Could you check a few things on this model? Use its own coordinates, in mm. Face numbers are marked on the shaded views. A direction names the side the tool comes from. Give positions to 0.01 mm unless a question says otherwise; leave off trailing zeros. Order: outer loops, then holes, each group sorted by start corner. A loop starts at its lowest first (then second) coordinate and runs counter-clockwise, first axis right, second up. Notation, with made-up numbers: M -34.5,17 L 22.5,17 A15 cw 22.5,31 Z; hole C 85.25,64.25 d10. An arc over 180 degrees is marked long. Answer in a Markdown table with one row per item. Add a question column.
```python
from build123d import *

# Parameters (mm, degrees)
PAD004_DEPTH    = 5
POCKET004_DEPTH = 2.001
PAD005_DEPTH    = 15
SKETCH015_R     = 1.55
POCKET005_DEPTH = 5.001
POCKET006_DEPTH = 2.65


with BuildPart() as part:
    # Sketch013 → Pad004 (new body)
    with BuildSketch(Plane.XY):
        with BuildLine():
            ThreePointArc((0, -7.5), (7.5, 0), (0, 7.5))
            Line((0, 7.5), (-40, 7.5))
            Line((-40, 7.5), (-40, 3.25))
            Line((0, 3.25), (-40, 3.25))
            ThreePointArc((0, -3.25), (3.25, 0), (0, 3.25))
            Line((0, -3.25), (-40, -3.25))
            Line((-40, -3.25), (-40, -7.5))
            Line((0, -7.5), (-40, -7.5))
        make_face()
    extrude(amount=PAD004_DEPTH)

    # Sketch012 → Pocket004 (cut, through all)
    with BuildSketch(Plane.XY.offset(3)):
        with BuildLine():
            ThreePointArc((0, -5.5), (5.5, 0), (0, 5.5))
            Line((0, 5.5), (-40, 5.5))
            ThreePointArc((-40, 5.5), (-45.5, 0), (-40, -5.5))
            Line((0, -5.5), (-40, -5.5))
        make_face()
    extrude(amount=POCKET004_DEPTH, mode=Mode.SUBTRACT)

    # Sketch014 → Pad005 (join)
    with BuildSketch(Plane.XZ.offset(7.5)):
        Polygon((-49, 5), (-50, 4), (-50, 1.3), (-40, 1.3), (-40, 0), (-39, 0), (-39, 5), (-40, 5), align=None)
    extrude(amount=-PAD005_DEPTH)

    # Sketch015 → Pocket005 (cut, through all)
    with BuildSketch(Plane.XY):
        with Locations((-44.5, 0)):
            Circle(SKETCH015_R)
    extrude(amount=POCKET005_DEPTH, mode=Mode.SUBTRACT)

    # Sketch016 → Pocket006 (cut)
    with BuildSketch(Plane.XY.offset(1.8)):
        Polygon((-44.5, 3.3), (-47.357884, 1.65), (-47.357884, -1.65), (-47.357884, -8.65), (-41.642116, -8.65), (-41.642116, -1.65), (-41.642116, 1.65), align=None)
    extrude(amount=POCKET006_DEPTH, mode=Mode.SUBTRACT)


solid = part.part
```
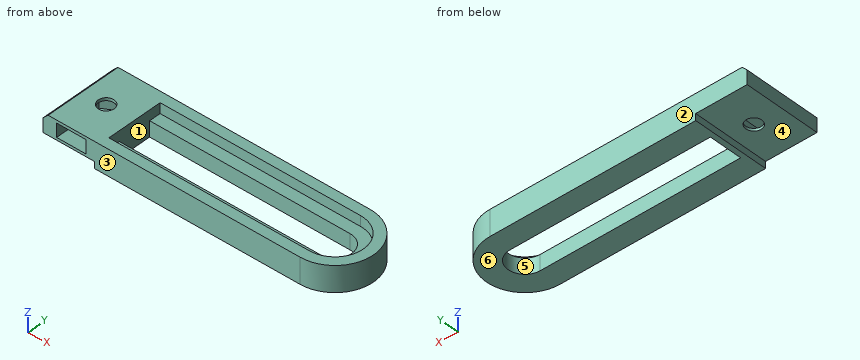
1. For the marked faces 4, 5 and 6, which set-ups out of +Z, -Z, +X, -X, +Y, -Y let a thin tool reach every point of the face, with its end or its side?
2. Suppose I cut it at A-A on x = -4. List the corners of the cut face in (y, z) for me, plus the area to 3 significant figures.
3. Suppose I cut it at B-B on y = 0. List the corners of the cut face in (x, z) for me, plus the area to 3 significant figures.
4. Thinking about a two-plate mould opening in Y: for the marked faces 1, 2 and 3, which applies, pulls with the +Y half, pulls with the -Y half, needs draft (parallel to the pull), parting line crosses it, or undercut?
5. If I drill on line 1 along Y through (x, z) = (-6.5, 3.45); line 2 along Y through (x, z) = (-44.5, 4.8); line 3 along X through (y, z) = (0, 4.85), over which ranges is the centre line in solid material (lowest first)? Write a range as [from, to].
6. Suppose I cut it at C-C on y = 4.75. List the corners of the cut face in (x, z) for me.
7. Will these pins go through, and if not, where does the flat tip stop? P1, Ø5, axis at x = -46.5, y = 3.5, coming from the -Z side; P2, Ø1.5, axis at y = 2.5, z = 3.5, coming from the +X side.
Findings below:
| question | item | result |
|---|---|---|
| 1 | face 4 | -Z, -X, +Y, -Y |
| 1 | face 5 | +Z, -Z |
| 1 | face 6 | -Z, +X, -X, +Y, -Y |
| 2 | outline | M -7.5,0 L -3.25,0 L -3.25,3 L -5.5,3 L -5.5,5 L -7.5,5 Z; M 3.25,0 L 7.5,0 L 7.5,5 L 5.5,5 L 5.5,3 L 3.25,3 Z |
| 2 | area | 33.5 mm2 |
| 3 | outline | M -50,1.3 L -46.05,1.3 L -46.05,1.8 L -47.36,1.8 L -47.36,4.45 L -46.05,4.45 L -46.05,5 L -49,5 L -50,4 Z; M -42.95,1.3 L -40,1.3 L -40,0 L -39,0 L -39,5 L -42.95,5 L -42.95,4.45 L -41.64,4.45 L -41.64,1.8 L -42.95,1.8 Z; M 3.25,0 L 7.5,0 L 7.5,5 L 5.5,5 L 5.5,3 L 3.25,3 Z |
| 3 | area | 39.8 mm2 |
| 4 | face 1 | undercut |
| 4 | face 2 | pulls with the +Y half |
| 4 | face 3 | pulls with the -Y half |
| 5 | line 1 | [-7.5, -5.5], [5.5, 7.5] |
| 5 | line 2 | [-7.5, -1.55], [1.55, 7.5] |
| 5 | line 3 | [-49.15, -46.05], [-42.95, -39], [5.5, 7.5] |
| 6 | outline | M -50,1.3 L -40,1.3 L -40,0 L 5.8,0 L 5.8,5 L 2.77,5 L 2.77,3 L -39,3 L -39,5 L -49,5 L -50,4 Z |
| 7 | P1 | z = 1.3 |
| 7 | P2 | x = 7.29 |
